```python
from build123d import *

# Parameters (mm, degrees)
SKETCH1_R           = 40
SKETCH1_R_2         = 30.5
BOSS_EXTRUDE1_DEPTH = 3
SKETCH2_W           = 42.273863656
SKETCH2_H           = 17
BOSS_EXTRUDE2_DEPTH = 3
SKETCH3_R           = 2.05
CUT_EXTRUDE1_DEPTH  = 4
FILLET1_R           = 3


with BuildPart() as part:
    # Sketch1 → Boss-Extrude1 (new body)
    with BuildSketch(Plane(origin=(0, 0, 0), x_dir=(1, 0, 0), z_dir=(0, 1, 0))):
        Circle(SKETCH1_R)
        Circle(SKETCH1_R_2, mode=Mode.SUBTRACT)
    extrude(amount=BOSS_EXTRUDE1_DEPTH)

    # Sketch2 → Boss-Extrude2 (add)
    with BuildSketch(Plane(origin=(0, 3, 0), x_dir=(1, 0, 0), z_dir=(0, 1, 0))):
        with Locations((53.863068172, 14.5)):
            Rectangle(SKETCH2_W, SKETCH2_H)
        with Locations((53.863068172, -14.5)):
            Rectangle(SKETCH2_W, SKETCH2_H)
    extrude(amount=-BOSS_EXTRUDE2_DEPTH)

    # Sketch3 → Cut-Extrude1 (cut, through all)
    with BuildSketch(Plane(origin=(0, 3, 0), x_dir=(1, 0, 0), z_dir=(0, 1, 0))):
        with Locations((53, 14.5)):
            Circle(SKETCH3_R)
        with Locations((68, 14.5)):
            Circle(SKETCH3_R)
        with Locations((53, -14.5)):
            Circle(SKETCH3_R)
        with Locations((68, -14.5)):
            Circle(SKETCH3_R)
    extrude(amount=-CUT_EXTRUDE1_DEPTH, mode=Mode.SUBTRACT)

    # Fillet1
    fillet1_edges = [part.edges().sort_by_distance(p)[0] for p in [
        (39.547439867, 1.5, -6),
        (32.726136344, 1.5, -23),
        (39.547439867, 1.5, 6),
        (32.726136344, 1.5, 23),
    ]]
    fillet(fillet1_edges, radius=FILLET1_R)


solid = part.part
```
Part model, mm, in its own coordinate system. A direction names the side the tool comes from. Round coordinates to 2 decimals unless told otherwise and drop trailing zeros. Loops run counter-clockwise (first coordinate to the right, second up) from the corner with the lowest first, then second, coordinate; pieces in that order, holes last. Notation, with made-up numbers: (77, -14.5) -> (87, -14.5) arc R18 cw to (87, -4.5) -> close; hole circle Ø11 at (51, 77.5). An arc over 180 degrees is marked (long way). Use one line per item in the form item = value. Start each with the question number.
Item 1: Two-plate mould, pull along X, no slides. Class faces 5 (the flat face through (75, 2, -14)), 6 (the cylindrical face through (50.95, 1.52, -14.59)), 7 (the cylindrical face through (51.373, 1.521, 15.747)), 8 (the flat face through (29.5, 0, -9.4)): released by +X, released by -X, zero draft, split by the parting line, or undercut.
Item 2: Band-saw the part on C-C (x = 49.5). List the corners of the cut face in (y, z).
Item 3: Band-saw the part on B-B (y = 0.8). List the corners of the cut face in (x, z), plus the area to 3 significant figures.
Item 4: Drill centre lines: line 1 along Z through (x, y) = (53, 1); line 2 along X through (y, z) = (1.4, -14.5); line 3 along X through (y, z) = (0.45, 13.5). Where is each one in solid material? Low to high.
Item 5: Band-saw the part on D-D (z = 26). List the corners of the cut face in (x, y), plus the area to 3 significant figures.
Item 6: Drop flat-ended pins along their axis: pin 1 Ø4.5 at (x, z) = (53, 14.5) entering from -Y; pin 2 Ø3.5 at (x, z) = (68, -14.5) entering from +Y. Give the stop position or say it passes through.
Item 7: Tool access for faces 1 (the flat face through (54, 2, -23)), 2 (the cylindrical face through (40.678, 1.479, 5.021)), 3 (the flat face through (54, 2, 23)), 4 (the flat face through (29.5, 3, -9.4)): list every direction of +Z, -Z, +X, -X, +Y, -Y with a clear straight run to the whole face (end or side of a thin tool).
Item 8: Band-saw the part on A-A (x = 68). List the corners of the cut face in (y, z), plus the area to 3 significant figures.
Data:
q1.face_5 = released by +X
q1.face_6 = undercut
q1.face_7 = undercut
q1.face_8 = zero draft
q2.outline = (0, -23) -> (3, -23) -> (3, -6) -> (0, -6) -> close; (0, 6) -> (3, 6) -> (3, 23) -> (0, 23) -> close
q3.outline = (31.86, -24.19) arc R3 cw to (34.25, -23) -> (75, -23) -> (75, -6) -> (42.9, -6) arc R3 cw to (39.9, -2.79) arc R40 ccw to (39.9, 2.79) arc R3 cw to (42.9, 6) -> (75, 6) -> (75, 23) -> (34.25, 23) arc R3 cw to (31.86, 24.19) arc R40 ccw (long way) to start; hole circle Ø61 at (0, 0); hole circle Ø4.1 at (53, -14.5); hole circle Ø4.1 at (53, 14.5); hole circle Ø4.1 at (68, -14.5); hole circle Ø4.1 at (68, 14.5)
q3.area = 3,350 mm^2
q4.line_1 = -23 to -16.55, -12.45 to -6, 6 to 12.45, 16.55 to 23
q4.line_2 = -37.28 to -26.83, 26.83 to 50.95, 55.05 to 65.95, 70.05 to 75
q4.line_3 = -37.65 to -27.35, 27.35 to 51.21, 54.79 to 66.21, 69.79 to 75
q5.outline = (-30.4, 0) -> (-15.95, 0) -> (-15.95, 3) -> (-30.4, 3) -> close; (15.95, 0) -> (30.4, 0) -> (30.4, 3) -> (15.95, 3) -> close
q5.area = 86.7 mm^2
q6.pin_1 = 0
q6.pin_2 = through
q7.face_1 = -Z, +X, +Y, -Y
q7.face_2 = +X, +Y, -Y
q7.face_3 = +Z, +X, +Y, -Y
q7.face_4 = +Z, -Z, +X, -X, +Y
q8.outline = (0, -23) -> (3, -23) -> (3, -16.55) -> (0, -16.55) -> close; (0, -12.45) -> (3, -12.45) -> (3, -6) -> (0, -6) -> close; (0, 6) -> (3, 6) -> (3, 12.45) -> (0, 12.45) -> close; (0, 16.55) -> (3, 16.55) -> (3, 23) -> (0, 23) -> close
q8.area = 77.4 mm^2
